For this review, take the finished solid that the model builds, in its own axes (mm). Round coordinates to 2 decimals unless told otherwise and drop trailing zeros. Loops run counter-clockwise (first coordinate to the right, second up) from the corner with the lowest first, then second, coordinate; pieces in that order, holes last. Notation, with made-up numbers: (-11, -5.5) -> (8, -5.5) arc R6 ccw to (8, 1.5) -> close; hole circle Ø6 at (49.5, 51.5). An arc over 180 degrees is marked (long way). One line per question, with ' | ' between items. Start each with the question number.
1. Consider section B-B (x = -6.25). Write out the cut boundary in (y, z).
2. Draft analysis for pull direction Y (two halves, no side actions). For faces 1 (the face through (0, 38, 20)), 2 (the face through (0, 85, 10)), 3 (the face through (0.14, 72.326, 10.521)), state which applies: pulls with the +Y half, pulls with the -Y half, needs draft (parallel to the pull), parting line crosses it, or undercut.
3. For pin 1 Ø5 at (x, z) = (5.5, 9.5) entering from -Y; pin 2 Ø3 at (x, z) = (3.5, 6) entering from +Y; pin 3 Ø1.5 at (x, z) = (-1, 9.5) entering from -Y, all flat-tipped, find the tip position at first contact; note any pin that passes through.
4. Consider section C-C (z = 12.5). Write out the cut boundary in (x, y), and give its area (3 significant figures).
5. Consider section A-A (y = 68.36). Write out the cut boundary in (x, z).
6. Wall thickness on line 1 along Y through (x, z) = (0, 10); line 2 along Y through (x, z) = (1.5, 10); line 3 along Y through (x, z) = (0.75, 16.25): over which ranges is each line inside the solid? List them lowest first.
7. Consider section D-D (y = 6.54). Write out the cut boundary in (x, z), and give its area (3 significant figures).
```python
from build123d import *

# Parameters (mm, degrees)
SKETCH2_R           = 5
BOSS_EXTRUDE1_DEPTH = 20
SKETCH4_R           = 4
CUT_EXTRUDE1_DEPTH  = 28
SKETCH5_R           = 5
CUT_EXTRUDE2_DEPTH  = 30
BOSS_EXTRUDE2_START = -20
SKETCH12_R          = 5
BOSS_EXTRUDE2_DEPTH = 20
SKETCH13_R          = 5
CUT_EXTRUDE3_DEPTH  = 20


with BuildPart() as part:
    # Sketch2 → Boss-Extrude1 (new body)
    with BuildSketch(Plane.XY):
        with BuildLine():
            Line((-10, 0), (-10, 75))
            ThreePointArc((-10, 75), (0, 85), (10, 75))
            Line((10, 75), (10, 0))
            ThreePointArc((10, 0), (0, -10), (-10, 0))
        make_face()
        Circle(SKETCH2_R, mode=Mode.SUBTRACT)
    extrude(amount=BOSS_EXTRUDE1_DEPTH)

    # Sketch4 → Cut-Extrude1 (cut)
    with BuildSketch(Plane(origin=(10, 0, 0), x_dir=(0, 0, -1), z_dir=(1, 0, 0))):
        with Locations((-10, 68.36)):
            Circle(SKETCH4_R)
    extrude(amount=-CUT_EXTRUDE1_DEPTH, mode=Mode.SUBTRACT)

    # Sketch5 → Cut-Extrude2 (cut)
    with BuildSketch(Plane(origin=(10, 0, 0), x_dir=(0, 0, -1), z_dir=(1, 0, 0))):
        with Locations((-10, 6.54)):
            Circle(SKETCH5_R)
    extrude(amount=-CUT_EXTRUDE2_DEPTH, mode=Mode.SUBTRACT)

    # Sketch12 → Boss-Extrude2 (add)
    with BuildSketch(Plane.XY.offset(20).offset(BOSS_EXTRUDE2_START)):
        Circle(SKETCH12_R)
    extrude(amount=BOSS_EXTRUDE2_DEPTH)

    # Sketch13 → Cut-Extrude3 (cut)
    with BuildSketch(Plane(origin=(10, 0, 0), x_dir=(0, 0, -1), z_dir=(1, 0, 0))):
        with Locations((-10, 6.54)):
            Circle(SKETCH13_R)
    extrude(amount=-CUT_EXTRUDE3_DEPTH, mode=Mode.SUBTRACT)


solid = part.part
```
Answer block:
1) outline: (-7.81, 0) -> (82.81, 0) -> (82.81, 20) -> (-7.81, 20) -> close; hole circle Ø10 at (6.54, 10); hole circle Ø8 at (68.36, 10)
2) face 1: needs draft | face 2: pulls with the +Y half | face 3: undercut
3) pin 1: stops at y = -9.54 | pin 2: stops at y = 84.8 | pin 3: stops at y = -10
4) outline: (-10, 0) arc R10 ccw to (10, 0) -> (10, 2.21) -> (-10, 2.21) -> close; (-10, 10.87) -> (10, 10.87) -> (10, 65.24) -> (-10, 65.24) -> close; (-10, 71.48) -> (10, 71.48) -> (10, 75) arc R10 ccw to (-10, 75) -> close | area: 1,520 mm2
5) outline: (-10, 0) -> (10, 0) -> (10, 6) -> (-10, 6) -> close; (-10, 14) -> (10, 14) -> (10, 20) -> (-10, 20) -> close
6) line 1: y = -10 to 1.54, 11.54 to 64.36, 72.36 to 85 | line 2: y = -9.89 to 1.54, 11.54 to 64.36, 72.36 to 84.89 | line 3: y = -9.97 to 84.97
7) outline: (-10, 0) -> (10, 0) -> (10, 5) -> (-10, 5) -> close; (-10, 15) -> (10, 15) -> (10, 20) -> (-10, 20) -> close | area: 200 mm2
